```python
from build123d import *

# Parameters (mm, degrees)
BOSS_EXTRUDE6_DEPTH = 0.2
BOSS_EXTRUDE8_DEPTH = 15.2
SKETCH2_W           = 50
SKETCH2_H           = 9
CUT_EXTRUDE1_DEPTH  = 2
SKETCH3_W           = 50
SKETCH3_H           = 9
CUT_EXTRUDE2_DEPTH  = 2
SKETCH4_W           = 50
SKETCH4_H           = 9
CUT_EXTRUDE3_DEPTH  = 2


with BuildPart() as part:
    # Sketch1 → Boss-Extrude6 (new body)
    with BuildSketch(Plane(origin=(0, 0, 0), x_dir=(1, 0, 0), z_dir=(0, 1, 0))):
        Polygon((351.272917769, 67.665499075), (468.273000096, -134.984588004), (464.273241085, -141.912373829), (230.273290915, -141.912373829), (226.272682949, -134.984246141), (343.272757546, 67.665499075), align=None)
    extrude(amount=BOSS_EXTRUDE6_DEPTH)

    # Sketch1<7> → Boss-Extrude8 (add)
    with BuildSketch(Plane(origin=(0, 0, 0), x_dir=(1, 0, 0), z_dir=(0, 1, 0))):
        Polygon((351.272917769, 67.665499075), (468.273000096, -134.984588004), (464.273241085, -141.912373829), (230.273290915, -141.912373829), (226.272682949, -134.984246141), (343.272757546, 67.665499075), align=None)
        Polygon((231.427991453, -139.912373829), (463.118576698, -139.912436444), (465.963671321, -134.984588004), (350.118252434, 65.665563332), (344.427420986, 65.665563332), (228.58200795, -134.984248572), align=None, mode=Mode.SUBTRACT)
    extrude(amount=BOSS_EXTRUDE8_DEPTH)

    # Sketch2 → Cut-Extrude1 (cut)
    with BuildSketch(Plane.XY.offset(141.912373829)):
        with Locations((344.427420986, 15.2)):
            Rectangle(SKETCH2_W, SKETCH2_H)
    extrude(amount=-CUT_EXTRUDE1_DEPTH, mode=Mode.SUBTRACT)

    # Sketch3 → Cut-Extrude2 (cut)
    with BuildSketch(Plane(origin=(292.754708906, 0, -169.022009994), x_dir=(-0.5000000000000001, 0, -0.8660254037844386), z_dir=(0.8660254037844386, 0, -0.5000000000000001))):
        with Locations((-234.036500052, 15.2)):
            Rectangle(SKETCH3_W, SKETCH3_H)
    extrude(amount=-CUT_EXTRUDE2_DEPTH, mode=Mode.SUBTRACT)

    # Sketch4 → Cut-Extrude3 (cut)
    with BuildSketch(Plane(origin=(228.154315179, 0, 131.7251688), x_dir=(-0.5000006078406093, 0, 0.866025052847215), z_dir=(-0.866025052847215, 0, -0.5000006078406093))):
        with Locations((-113.236672478, 15.2)):
            Rectangle(SKETCH4_W, SKETCH4_H)
    extrude(amount=-CUT_EXTRUDE3_DEPTH, mode=Mode.SUBTRACT)


solid = part.part
```
Design review of the part built by this model. Coordinates are the model's own, in mm. A direction names the side the tool comes from. Coordinates: 2 decimals unless noted, no trailing zeros. Loops run counter-clockwise (first coordinate to the right, second up) from the corner with the lowest first, then second, coordinate; pieces in that order, holes last. Notation, with made-up numbers: M -37,72.5 L 12,72.5 A29 cw 12,105.5 Z; hole C -24,31 d4. An arc over 180 degrees is marked long. One line per question, with ' | ' between items.
(1) We need section B-B (z = 23). Give the boundary of the cut face in (x, y), and give its area (3 significant figures).
Filled in:
outline: M 290.93,0 L 403.62,0 L 403.62,10.7 L 401.31,10.7 L 401.31,0.2 L 293.24,0.2 L 293.24,10.7 L 290.93,10.7 Z | area: 71.0 mm^2
(2) We need section A-A (y = 6). Give the boundary of the cut face in (x, z), and give its area (3 significant figures).
Filled in:
outline: M 226.27,134.98 L 343.27,-67.67 L 351.27,-67.67 L 468.27,134.98 L 464.27,141.91 L 230.27,141.91 Z; hole M 228.58,134.98 L 344.43,-65.67 L 350.12,-65.67 L 465.96,134.98 L 463.12,139.91 L 231.43,139.91 Z | area: 1,440 mm^2
(3) Wall thickness on probe 1 along Y at (x, z) = (247, 120.5); probe 2 along Z at (x, y) = (357.5, 7.5); probe 3 along Z at (x, y) = (359, 9): over which ranges is each line inside the solid? List them lowest first.
Filled in:
probe 1: y = 0 to 0.2 | probe 2: z = -56.88 to -52.88, 139.91 to 141.91 | probe 3: z = -54.28 to -50.28, 139.91 to 141.91
(4) We need section C-C (x = 338.5). Give the boundary of the cut face in (y, z).
Filled in:
outline: M 0,-59.4 L 15.2,-59.4 L 15.2,-55.4 L 0.2,-55.4 L 0.2,139.91 L 10.7,139.91 L 10.7,141.91 L 0,141.91 Z
(5) Draft analysis for pull direction Z (two halves, no side actions). For faces 3 (the face through (262.7, 15.2, 140.1)), 4 (the face through (408.954, 7.494, 32.241)), 5 (the face through (464.521, 7.595, 137.483)), state which applies: released by +Z, released by -Z, zero draft, split by the parting line, or undercut.
Filled in:
face 3: zero draft | face 4: released by -Z | face 5: undercut
(6) For pin 1 Ø2 at (y, z) = (12.5, 141.5) entering from -X; pin 2 Ø1.6 at (y, z) = (12.5, 140.5) entering from +X; pin 3 Ø8 at (x, z) = (288, 41) entering from +Y, all flat-tipped, find the tip position at first contact; note any pin that passes through.
Filled in:
pin 1: stops at x = 229.46 | pin 2: stops at x = 465.55 | pin 3: stops at y = 0.2
(7) Machinability: for faces 1 (the face through (426.4, 15.2, 140.1)), 2 (the face through (287.32, 7.59, 33.25)), which of the approach directions +Z, -Z, +X, -X, +Y, -Y give a long, thin tool a straight path to every point of the face, cutting with its end or side? Answer none if there is none.
Filled in:
face 1: +Z, -Z, +X, -X, +Y | face 2: +Y
